```python
from build123d import *

# Parameters (mm, degrees)
SKETCH1_R                     = 23
SKETCH1_R_2                   = 10
BOSS_EXTRUDE1_DEPTH           = 4
CHAMFER1_SIZE                 = 0.5
CHAMFER2_SIZE                 = 1
CSK_FOR_M3_SFHCS1_D           = 3.4
CSK_FOR_M3_SFHCS1_CSINK_D     = 6.72
CSK_FOR_M3_SFHCS1_CSINK_ANGLE = 90


with BuildPart() as part:
    # Sketch1 → Boss-Extrude1 (new body)
    with BuildSketch(Plane(origin=(0, 0, 0), x_dir=(1, 0, 0), z_dir=(0, 1, 0))):
        with Locations(Location((0, 0, 0), (0, 0, 270))):
            Circle(SKETCH1_R)
        with Locations(Location((0, 0, 0), (0, 0, 270))):
            Circle(SKETCH1_R_2, mode=Mode.SUBTRACT)
    extrude(amount=BOSS_EXTRUDE1_DEPTH)

    # Chamfer1
    chamfer1_edges = [part.edges().sort_by_distance(p)[0] for p in [
        (0, 0, -10),
        (0, 4, -10),
    ]]
    chamfer(chamfer1_edges, length=CHAMFER1_SIZE)

    # Chamfer2
    chamfer2_edges = [part.edges().sort_by_distance(p)[0] for p in [
        (0, 4, -23),
    ]]
    chamfer(chamfer2_edges, length=CHAMFER2_SIZE)

    # CSK for M3 SFHCS1 (through all)
    with Locations(Plane(origin=(0, 4, 0), x_dir=(1, 0, 0), z_dir=(0, 1, 0))):
        with Locations((0, 19), (16.454482672, -9.5), (-16.454482672, -9.5)):
            CounterSinkHole(CSK_FOR_M3_SFHCS1_D / 2, CSK_FOR_M3_SFHCS1_CSINK_D / 2, counter_sink_angle=CSK_FOR_M3_SFHCS1_CSINK_ANGLE)


solid = part.part
```
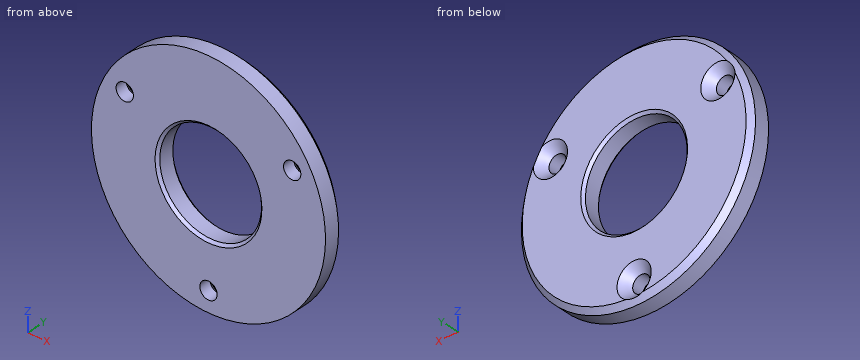
Could you check a few things on this model? Use its own coordinates, in mm. Coordinates: 2 decimals unless noted, no trailing zeros. Write each loop counter-clockwise with the first axis right and the second up, starting at its lowest first coordinate (ties: lowest second). Pieces come first, ordered by that corner, then holes. Notation, with made-up numbers: (44, 66.25) - (66, 66.25) arc R31 cw to (66, 93.25) - close; hole circle Ø9 at (23.5, -25). An arc over 180 degrees is marked (long way). Use a Markdown table: item, result.
Q1. Imagine slicing it at A-A (x = 0). List the corners of the cut face in (y, z) for me.
Geometry check:
| item | result |
|---|---|
| outline | (0, -23) - (3, -23) - (3.82, -22.18) - (2.34, -20.7) - (0, -20.7) - close; (0, -17.3) - (2.34, -17.3) - (4, -15.64) - (4, -10.5) - (3.5, -10) - (0.5, -10) - (0, -10.5) - close; (0, 10.5) - (0.5, 10) - (3.5, 10) - (4, 10.5) - (4, 22) - (3, 23) - (0, 23) - close |
Q2. Imagine slicing it at C-C (y = 1.6). List the corners of the cut face in (x, z) for me, and give its area (3 significant figures).
Geometry check:
| item | result |
|---|---|
| outline | circle Ø46 at (0, 0); hole circle Ø3.4 at (-16.45, 9.5); hole circle Ø20 at (0, 0); hole circle Ø3.4 at (0, -19); hole circle Ø3.4 at (16.45, 9.5) |
| area | 1,320 mm2 |
Q3. Imagine slicing it at B-B (z = 0). List the corners of the cut face in (x, y) for me, and give its area (4 significant figures).
Geometry check:
| item | result |
|---|---|
| outline | (-23, 0) - (-10.5, 0) - (-10, 0.5) - (-10, 3.5) - (-10.5, 4) - (-22, 4) - (-23, 3) - close; (10, 0.5) - (10.5, 0) - (23, 0) - (23, 3) - (22, 4) - (10.5, 4) - (10, 3.5) - close |
| area | 102.5 mm2 |
Q4. I'm going to push a flat-ended pin straight in: pin 1 Ø2 at (x, z) = (-16.45, 9.5) entering from +Y. Where does the tip first touch, or does it pass through?
Geometry check:
| item | result |
|---|---|
| pin 1 | passes through |
Q5. Please list where these lines run through material, in increasing order: L1, parallel to X at y = 1.05, z = 8; L2, parallel to X at y = 2.85, z = 0; L3, parallel to X at y = 2.7, z = -2.
Geometry check:
| item | result |
|---|---|
| L1 | x = -21.56 to -17.25, -15.65 to -6, 6 to 15.65, 17.25 to 21.56 |
| L2 | x = -23 to -10, 10 to 23 |
| L3 | x = -22.91 to -9.8, 9.8 to 22.91 |
